Autodesk Inventor part; units mm, degrees
ref_plane "YZ Plane" through (0, 0, 0) normal (1, 0, 0) x (0, 1, 0)
ref_plane "XZ Plane" through (0, 0, 0) normal (0, 1, 0) x (-1, 0, 0)
ref_plane "XY Plane" through (0, 0, 0) normal (0, 0, 1) x (1, 0, 0)
sketch "Эскиз1" plane through (0, 0, 0) normal (0, 1, 0) x (-1, 0, 0)
  line L0 (0, 0) -> (3, 0)
  line L1 (3, 0) -> (3, -3)
  line L2 (3, -3) -> (0, -3)
  line L3 (0, -3) -> (0, 0)
  line L4 (3, 0) -> (20, 0)
  line L5 (20, 0) -> (17, 0)
  line L6 (17, 0) -> (17, -3)
  line L7 (17, -3) -> (20, -3)
  line L8 (20, -3) -> (20, 0)
  line L9 (20, 0) -> (37, 0)
  line L10 (37, 0) -> (34, 0)
  line L11 (34, 0) -> (34, -3)
  line L12 (34, -3) -> (37, -3)
  line L13 (37, -3) -> (37, 0)
  line L14 (37, 0) -> (54, 0)
  line L15 (54, 0) -> (51, 0)
  line L16 (51, 0) -> (51, -3)
  line L17 (51, -3) -> (54, -3)
  line L18 (54, -3) -> (54, 0)
  point P0 (17, 0)
  point P1 (17, 0)
  dimension "d0" = 3
  dimension "d1" = 3
  dimension "d17" = 17
  dimension "d18" = 3
  dimension "d19" = 3
  dimension "d20" = 17
  dimension "d21" = 17
  dimension "d22" = 3
  dimension "d23" = 3
  dimension "d24" = 3
  dimension "d25" = 3
extrude "Выдавливание1" add sketch "Эскиз1" along normal blind 4
sketch "Эскиз2" plane through (0, 4, 0) normal (0, 1, 0) x (1, 0, 0)
  line L0 (0, 0) -> (-100, 0)
  line L1 (-100, 0) -> (-100, 3)
  line L2 (-100, 3) -> (0, 3)
  line L3 (0, 3) -> (0, 0)
  dimension "d13" = 3
  dimension "d14" = 100
extrude "Выдавливание2" add sketch "Эскиз2" along normal blind 15
fillet "Сопряжение1" radius 1 1 edges at (-17, 4, -1.5)
fillet "Сопряжение2" radius 2 7 edges at (-34, 4, -1.5) (-51, 4, -1.5) (-54, 4, -1.5) (-37, 4, -1.5) (-20, 4, -1.5) (-3, 4, -1.5) (0, 19, -1.5)
fillet "Сопряжение3" radius 2 2 edges at (-100, 19, -1.5) (-100, 4, -1.5)
sketch "Эскиз3" plane through (-54, 0, 0) normal (0, 0, 1) x (1, 0, 0)
  line L0 (-46, 6) -> (-46, 17)
  circle A0 centre (-41, 11.5) radius 2.5
  line L1 (-46, 15.899) -> (-46, 11.5)
  point P0 (54, 0)
  dimension "d30" = 5
extrude "Выдавливание3" cut sketch "Эскиз3" against normal blind 14
properties part number "Bus_copper_VDD" material "Медь"
Design review of the part built by this model. Coordinates are the model's own, in mm. A direction names the side the tool comes from. Coordinates: 2 decimals unless noted, no trailing zeros. Loops run counter-clockwise (first coordinate to the right, second up) from the corner with the lowest first, then second, coordinate; pieces in that order, holes last. Notation, with made-up numbers: (84.25, -8) -> (142.25, -8) arc R23 ccw to (142.25, 18) -> close; hole circle Ø9 at (42.25, -10). An arc over 180 degrees is marked (long way). Answer as a JSON object with one key per item and string values.
Q1. Tool access review of faces 1 (the flat face through (0, 8, -2)), 2 (the flat face through (-17, 1, -1)), 3 (the flat face through (-54, 1, -2)): name each direction out of +Z, -Z, +X, -X, +Y, -Y from which nothing blocks a thin tool from reaching the whole face with its end or side.
Answer block:
{"face 1": "+Z, -Z, +X, +Y, -Y", "face 2": "+Z, -Z, -Y", "face 3": "+Z, -Z, -X, -Y"}
Q2. To check wall thickness, follow L1, parallel to X at y = 1.5, z = -1.25; L2, parallel to Y at x = -95, z = -1.2; L3, parallel to Y at x = -57.5, z = -1.45. State the ranges of each line that lie inside material, in increasing order.
Answer block:
{"L1": "x = -54 to -51, -37 to -34, -20 to -17, -3 to 0", "L2": "y = 4 to 9, 14 to 19", "L3": "y = 4 to 19"}
Q3. Take a section at B-B on x = -95. Give the boundary of the cut face in (y, z).
Answer block:
{"outline": "(4, -3) -> (9, -3) -> (9, 0) -> (4, 0) -> close; (14, -3) -> (19, -3) -> (19, 0) -> (14, 0) -> close"}
Q4. The part is to be moulded in two halves that separate along X. For faces 4 (the cylindrical face through (-54.57, 3.4, -1.48)), 5 (the flat face through (-27, 4, -2)), 6 (the flat face through (-51, 19, -2)), say which applies: +X half, -X half, draft (parallel to the pull), parting line (faces both ways), or undercut.
Answer block:
{"face 4": "-X half", "face 5": "undercut", "face 6": "draft"}
Q5. Take a section at C-C on y = 11.5. Give the boundary of the cut face in (x, z), plus the area to 3 significant figures.
Answer block:
{"outline": "(-100, -3) -> (-97.5, -3) -> (-97.5, 0) -> (-100, 0) -> close; (-92.5, -3) -> (0, -3) -> (0, 0) -> (-92.5, 0) -> close", "area": "285 mm^2"}
Q6. Take a section at D-D on x = -23. Give the boundary of the cut face in (y, z).
Answer block:
{"outline": "(4, -3) -> (19, -3) -> (19, 0) -> (4, 0) -> close"}
Q7. Clearance check with flat-ended pins moving along their axes: pin 1 Ø1.5 at (x, z) = (-78, -2.5) entering from -Y; pin 2 Ø4 at (x, y) = (-95, 11.5) entering from +Z; pin 3 Ø1.6 at (y, z) = (0.5, -1) entering from -X. State where each tip first meets the part, or that it passes through.
Answer block:
{"pin 1": "stops at y = 4", "pin 2": "passes through", "pin 3": "stops at x = -54"}
